```python
from build123d import *

# Parameters (mm, degrees)
F0_W     = 0.2
F0_H     = 10
F0_W_2   = 0.3
F0_W_3   = 0.4
F0_W_4   = 0.5
F0_W_5   = 0.6
F0_W_6   = 0.7
F0_W_7   = 0.8
F0_W_8   = 0.9
F0_W_9   = 1
F0_W_10  = 1.1
F0_W_11  = 1.2
F1_DEPTH = 10
F2_W     = 67.7
F2_H     = 3.33333
F3_DEPTH = 10.001
F4_W     = 67.7
F4_H     = 10
F4_W_2   = 63.7
F4_H_2   = 2
F5_DEPTH = 0.4


with BuildPart() as f1:
    # F0 (on Top) → F1 (new body)
    with BuildSketch(Plane.XY):
        with Locations((5.1, 0)):
            Rectangle(F0_W, F0_H)
        with Locations((6.35, 0)):
            Rectangle(F0_W_2, F0_H)
        with Locations((8.7, 0)):
            Rectangle(F0_W_3, F0_H)
        with Locations((12.15, 0)):
            Rectangle(F0_W_4, F0_H)
        with Locations((16.7, 0)):
            Rectangle(F0_W_5, F0_H)
        with Locations((22.35, 0)):
            Rectangle(F0_W_6, F0_H)
        with Locations((29.1, 0)):
            Rectangle(F0_W_7, F0_H)
        with Locations((36.95, 0)):
            Rectangle(F0_W_8, F0_H)
        with Locations((45.9, 0)):
            Rectangle(F0_W_9, F0_H)
        with Locations((55.95, 0)):
            Rectangle(F0_W_10, F0_H)
        with Locations((67.1, 0)):
            Rectangle(F0_W_11, F0_H)
    extrude(amount=F1_DEPTH)

    # F2 (on Top) → F3 (cut, through all)
    with BuildSketch(Plane.XY):
        with Locations((33.85, 0)):
            Rectangle(F2_W, F2_H)
    extrude(amount=F3_DEPTH, mode=Mode.SUBTRACT)

    # F4 (on Top) → F5 (join)
    with BuildSketch(Plane.XY):
        with Locations((33.85, 0)):
            Rectangle(F4_W, F4_H)
        with Locations((33.85, 0)):
            Rectangle(F4_W_2, F4_H_2, mode=Mode.SUBTRACT)
    extrude(amount=F5_DEPTH)


solid = f1.part
```
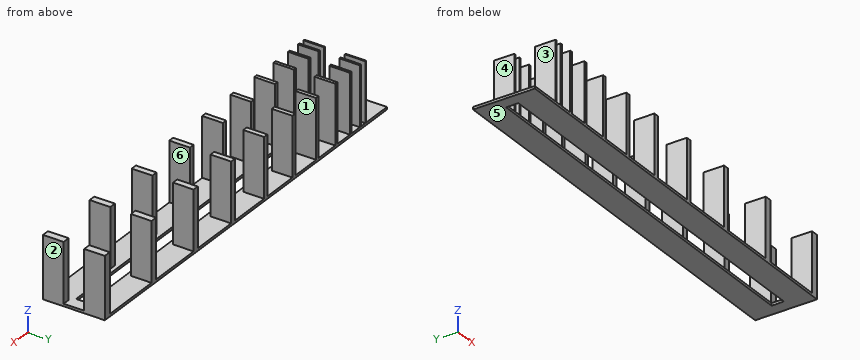
Can you work these out from the model? Positions are in its coordinate system, mm. Face numbers are marked on the shaded views. A direction names the side the tool comes from. Coordinates: 2 decimals unless noted, no trailing zeros. Order: outer loops, then holes, each group sorted by start corner. A loop starts at its lowest first (then second) coordinate and runs counter-clockwise, first axis right, second up.
1. If we section it at C-C (z = 5.5): Give the number of separate pieces and of enclosed holes in the cut face, then the cut area to 3 significant figures.
2. If we section it at A-A (x = 33.5): Please give me the cut outline in (y, z).
3. For the marked faces 4, 5 and 6, which set-ups out of +Z, -Z, +X, -X, +Y, -Y let a thin tool reach every point of the face, with its end or its side?
4. I need wall thicknesses on line 1 (Y direction, x = 12, z = 2.25); line 2 (Z direction, x = 53, y = 3). Which ranges of each line are inside material? Lowest first, please.
5. Thinking about a two-plate mould opening in X: for the marked faces 1, 2 and 3, which applies, +X half, -X half, draft (parallel to the pull), parting line (faces both ways), or undercut?
6. I'm going to push flat-ended pins straight in: pin 1 (1.5 mm diameter, centred on x = 60, z = 3, fed in from +Y); pin 2 (2.5 mm diameter, centred on y = -3, z = 4, fed in from -X). Where does each tip first touch, or does it pass through?
7. If we section it at B-B (y = -0.25): Please give me the cut outline in (x, z), then the cut area to 3 significant figures.
Entries:
1. separate pieces: 22
1. enclosed holes: 0
1. area: 51.3 mm2
2. outline: (-5, 0) - (-1, 0) - (-1, 0.4) - (-5, 0.4) - close; (1, 0) - (5, 0) - (5, 0.4) - (1, 0.4) - close
3. face 4: +Z, -X, +Y, -Y
3. face 5: -Z, +X, -X, +Y, -Y
3. face 6: +Z, +Y, -Y
4. line 1: y = -5 to -1.67, 1.67 to 5
4. line 2: z = 0 to 0.4
5. face 1: undercut
5. face 2: +X half
5. face 3: -X half
6. pin 1: passes through
6. pin 2: stops at x = 5
7. outline: (0, 0) - (2, 0) - (2, 0.4) - (0, 0.4) - close; (65.7, 0) - (67.7, 0) - (67.7, 0.4) - (65.7, 0.4) - close
7. area: 1.60 mm2
